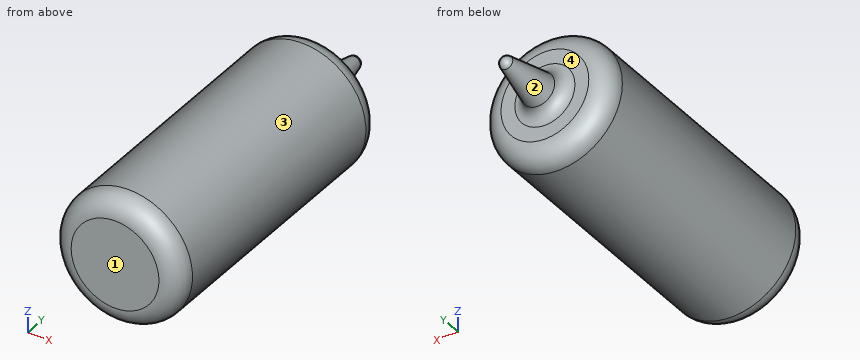
Autodesk Inventor part; units mm, degrees
ref_plane "YZ Plane" through (0, 0, 0) normal (1, 0, 0) x (0, 1, 0)
ref_plane "XZ Plane" through (0, 0, 0) normal (0, 1, 0) x (-1, 0, 0)
ref_plane "XY Plane" through (0, 0, 0) normal (0, 0, 1) x (1, 0, 0)
sketch "Sketch1" plane through (0, 0, 0) normal (0, 0, 1) x (1, 0, 0)
  line L0 (0, 0) -> (-6.5, 0)
  line L1 (-9.5, 3) -> (-9.5, 42)
  arc A0 (0, 54.5) -> (-0.9781, 53.7079) centre (0, 53.5) ccw
  line L2 (-0.9781, 53.7079) -> (-2.4923, 46.5842)
  line L3 (-6.5, 45) -> (-4.4486, 45)
  arc A1 (-4.4486, 45) -> (-2.4923, 46.5842) centre (-4.4486, 47) ccw
  arc A2 (-6.5, 45) -> (-9.5, 42) centre (-6.5, 42) ccw
  arc A3 (-9.5, 3) -> (-6.5, 0) centre (-6.5, 3) ccw
  line L4 (0, 63.3885) -> (0, -6.2417)
  point P0 (0, 0)
  dimension "d0" = 2
  dimension "d1" = 3
  dimension "d2" = 45
  dimension "d3" = 1
  dimension "d5" = 53.5
  dimension "d7" = 12
  dimension "d8" = 19
revolve "Revolution1" add sketch "Sketch1" angle 360 about axis through (0, 63.3885, 0) along (0, -1, 0)
properties part number "IN-14"
Geometry check sheet. Reference: the model listing, model coordinates, mm. Face numbers are marked on the shaded views. A direction names the side the tool comes from. Give positions to 0.01 mm unless a question says otherwise; leave off trailing zeros. Loops run counter-clockwise (first coordinate to the right, second up) from the corner with the lowest first, then second, coordinate; pieces in that order, holes last. Notation, with made-up numbers: (49, 42.5) -> (82, 42.5) arc R22 cw to (82, 67.5) -> close; hole circle Ø3 at (0, -37.75). An arc over 180 degrees is marked (long way). Answer in a Markdown table with one row per item. Add a question column.
1) Gauge pin test, flat ends, axial feed: P1, Ø10, axis at y = 5.5, z = 6.5, coming from the -X side; P2, Ø6, axis at x = -6.5, y = 33, coming from the +Z side; P3, Ø1.5, axis at y = 36.5, z = -2, coming from the +X side. Record the tip position at first contact, or that the pin passes through.
2) Set-up check for the marked faces 3 and 4: record each of +Z, -Z, +X, -X, +Y, -Y from which the full face is reachable in a straight line by a thin tool's end or side.
3) Material ranges on probe 1 along Y at (x, z) = (-0.25, -6); probe 2 along X at (y, z) = (47, 1.5); probe 3 along Y at (x, z) = (-5.75, 7), recorded low to high. Write a range as from..to.
4) Cross-section at A-A on y = 24.5. Record the boundary of the cut face in (x, z).
5) Draft check along X on the marked faces 1 and 2. Enter one of: pulls with the +X half, pulls with the -X half, needs draft (parallel to the pull), parting line crosses it, or undercut.
Outcome:
| question | item | result |
|---|---|---|
| 1 | P1 | stops at x = -9.38 |
| 1 | P2 | stops at z = 8.83 |
| 1 | P3 | stops at x = 9.42 |
| 2 | face 3 | +Y, -Y |
| 2 | face 4 | +Y |
| 3 | probe 1 | y = 0..45 |
| 3 | probe 2 | x = -1.88..1.88 |
| 3 | probe 3 | y = 1.43..43.57 |
| 4 | outline | circle Ø19 at (0, 0) |
| 5 | face 1 | needs draft |
| 5 | face 2 | parting line crosses it |
